Design review of the part shown in the three views and the two pictorial views. Dimensions are in mm from the part's minimum x, y and z. A direction names the side the tool comes from. Round coordinates to 2 decimals unless told otherwise and drop trailing zeros. Write each loop counter-clockwise with the first axis right and the second up, starting at its lowest first coordinate (ties: lowest second). Pieces come first, ordered by that corner, then holes. Notation, with made-up numbers: (-23, 10.5) -> (24, 10.5) arc R30 ccw to (24, 37.5) -> close; hole circle Ø2 at (17, 46.25). An arc over 180 degrees is marked (long way). Answer as a JSON object with one key per item and string values. Group by question number.
1) We need section B-B, the plane x = 7. Write out the cut boundary in (y, z).
2) Insertion check: pin 1 Ø1 at (x, y) = (20.5, 3) entering from +Z; pin 2 Ø1.6 at (x, y) = (11.5, 6) entering from -Z; pin 3 Ø1.1 at (x, z) = (18.5, 1.5) entering from -Y. Each pin has a flat end and moves straight along its axis. Give the tip position at first contact, or say it passes through.
3) We need section A-A, the plane y = 6. Write out the cut boundary in (x, z), then the cut area to 3 significant figures.
4) To check wall thickness, follow probe 1 along X at (y, z) = (6, 0.45); probe 2 along X at (y, z) = (4, 3.1); probe 3 along Y at (x, z) = (3.5, 3.15). State the ranges of each line that lie inside material, in increasing order. Write a range as [from, to].
5) Machinability: for the marked faces 1 and 2, which of the approach directions +Z, -Z, +X, -X, +Y, -Y give a long, thin tool a straight path to every point of the face, cutting with its end or side? Answer none if there is none.
6) We need section D-D, the plane y = 3.5. Write out the cut boundary in (x, z), then the cut area to 3 significant figures.
7) Mouldability with a two-part tool opening along Z and no side actions: class the marked faces 3, 4 and 5 as pulls with the +Z half, pulls with the -Z half, needs draft (parallel to the pull), parting line crosses it, or undercut.
8) We need section C-C, the plane z = 1.55. Write out the cut boundary in (x, y).
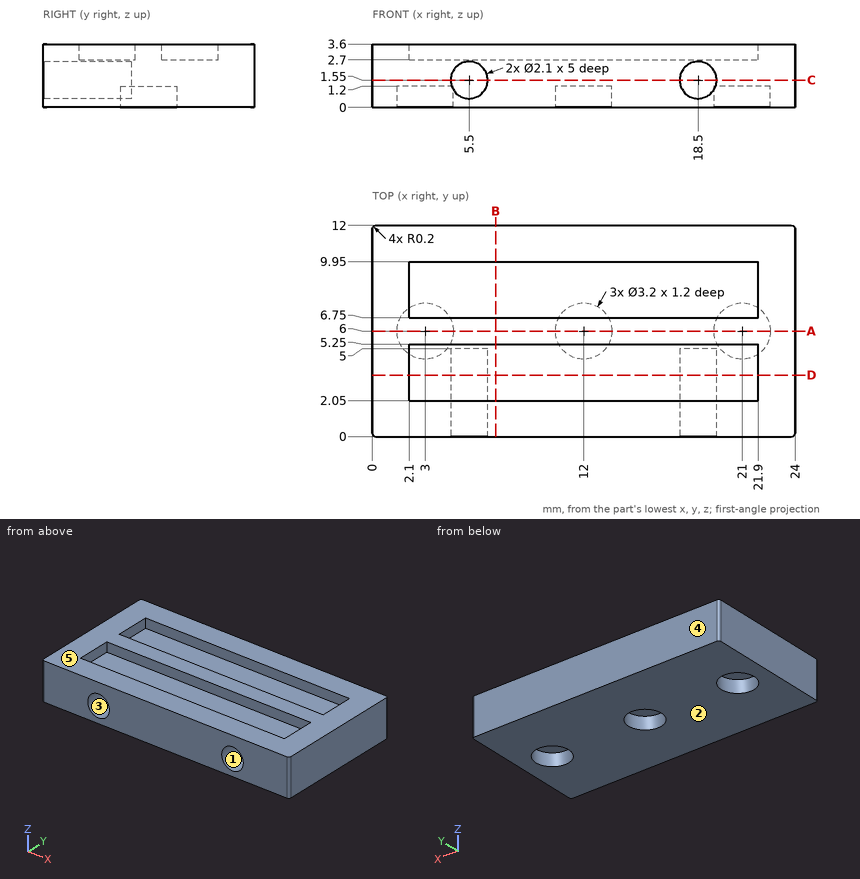
Here are the results:
{
 "1": {"outline": "(0, 0) -> (12, 0) -> (12, 3.6) -> (9.95, 3.6) -> (9.95, 2.7) -> (6.75, 2.7) -> (6.75, 3.6) -> (5.25, 3.6) -> (5.25, 2.7) -> (2.05, 2.7) -> (2.05, 3.6) -> (0, 3.6) -> close"},
 "2": {"pin 1": "stops at z = 2.7", "pin 2": "stops at z = 1.2", "pin 3": "stops at y = 5"},
 "3": {"outline": "(0, 0) -> (1.4, 0) -> (1.4, 1.2) -> (4.6, 1.2) -> (4.6, 0) -> (10.4, 0) -> (10.4, 1.2) -> (13.6, 1.2) -> (13.6, 0) -> (19.4, 0) -> (19.4, 1.2) -> (22.6, 1.2) -> (22.6, 0) -> (24, 0) -> (24, 3.6) -> (0, 3.6) -> close", "area": "74.9 mm^2"},
 "4": {"probe 1": "x = [0, 1.4], [4.6, 10.4], [13.6, 19.4], [22.6, 24]", "probe 2": "x = [0, 2.1], [21.9, 24]", "probe 3": "y = [0, 2.05], [5.25, 6.75], [9.95, 12]"},
 "5": {"face 1": "-Y", "face 2": "-Z, +X, -X, +Y, -Y"},
 "6": {"outline": "(0, 0) -> (24, 0) -> (24, 3.6) -> (21.9, 3.6) -> (21.9, 2.7) -> (2.1, 2.7) -> (2.1, 3.6) -> (0, 3.6) -> close; hole circle Ø2.1 at (5.5, 1.55); hole circle Ø2.1 at (18.5, 1.55)", "area": "61.7 mm^2"},
 "7": {"face 3": "undercut", "face 4": "needs draft", "face 5": "pulls with the +Z half"},
 "8": {"outline": "(0, 0.2) arc R0.2 ccw to (0.2, 0) -> (4.45, 0) -> (4.45, 5) -> (6.55, 5) -> (6.55, 0) -> (17.45, 0) -> (17.45, 5) -> (19.55, 5) -> (19.55, 0) -> (23.8, 0) arc R0.2 ccw to (24, 0.2) -> (24, 11.8) arc R0.2 ccw to (23.8, 12) -> (0.2, 12) arc R0.2 ccw to (0, 11.8) -> close"}
}
